Source: CAD feature listing. Evaluate the final solid. Frame: model axes, mm. Face numbers are marked on the shaded views. Round coordinates to 2 decimals unless told otherwise and drop trailing zeros. Loops run counter-clockwise (first coordinate to the right, second up) from the corner with the lowest first, then second, coordinate; pieces in that order, holes last. Notation, with made-up numbers: (8.25, 10) - (49.25, 10) arc R17 ccw to (49.25, 23) - close; hole circle Ø3 at (75, 87.25). An arc over 180 degrees is marked (long way). One line per question, with ' | ' between items. Start each with the question number.
1. Ray query, line 1 (Y direction, x = 12, z = 278.5); line 2 (X direction, y = 19, z = 761.5); line 3 (X direction, y = 4.3, z = 390). Return the intervals inside material, ascending.
2. Cut plane A-A (x = 25). Return loops of the section in (y, z), then the cut area to 3 significant figures.
3. Cut plane C-C (y = 57). Return loops of the section in (x, z) (3 decimals), then the cut area to 3 significant figures.
4. Cut plane D-D (z = 1113.5). Return loops of the section in (x, y).
5. Mould query, pull axis X, two halves, no side actions, for the marked faces 1 and 2. Classes: pulls with the +X half, pulls with the -X half, needs draft (parallel to the pull), parting line crosses it, or undercut.
6. Cut plane B-B (z = 303). Return loops of the section in (x, y), then the cut area to 3 significant figures.
7. Pin query (flat end, axial travel): pin 1 (4 mm diameter, centred on x = 10, z = 354, fed in from -Y); pin 2 (1 mm diameter, centred on y = 2.5, z = 469.5, fed in from -X); pin 3 (10 mm diameter, centred on y = -6, z = 932, fed in from +X); pin 4 (3 mm diameter, centred on x = 39, z = 341.5, fed in from -Y). Return the tip coordinate at first contact, or that it passes through.
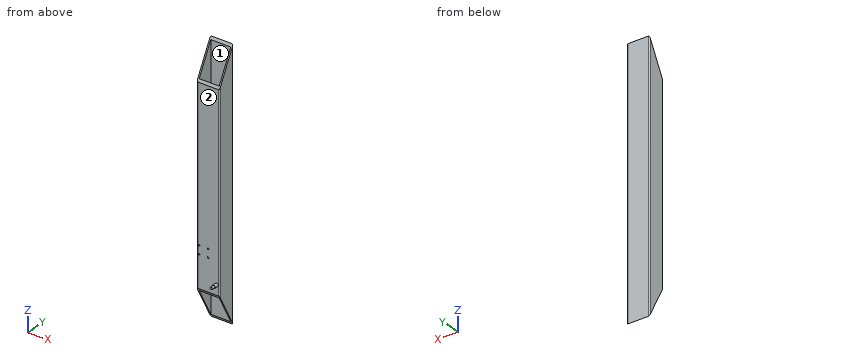
```python
from build123d import *

# Parameters (mm, degrees)
SCHIZZO1_W                   = 88
SCHIZZO1_H                   = 68
ESTRUSIONE_SOTTILE1_DEPTH    = 1200
ESTRUSIONE1_DEPTH            = 1207.813987324
SCHIZZO3_R                   = 3.4
TAGLIO_ESTRUSIONE1_DEPTH     = 10
RIPETIZIONE_A_L1_COUNT       = 2
RIPETIZIONE_A_L1_PITCH       = 40
RIPETIZIONE_A_L1_COUNT_DIR2  = 2
RIPETIZIONE_A_L1_PITCH_DIR2  = 36
SCHIZZO4_R                   = 7
ESTRUSIONE_ESTRUSIONE1_DEPTH = 18
SCHIZZO5_R                   = 5
ESTRUSIONE_ESTRUSIONE2_DEPTH = 15


with BuildPart() as part:
    # Schizzo1 → Estrusione-Sottile1 (new body)
    with BuildSketch(Plane.XY):
        with BuildLine():
            Line((5, 0), (95, 0))
            ThreePointArc((95, 0), (98.535533906, 1.464466094), (100, 5))
            Line((100, 5), (100, 75))
            ThreePointArc((100, 75), (98.535533906, 78.535533906), (95, 80))
            Line((95, 80), (5, 80))
            ThreePointArc((5, 80), (1.464466094, 78.535533906), (0, 75))
            Line((0, 75), (0, 5))
            ThreePointArc((0, 5), (1.464466094, 1.464466094), (5, 0))
        make_face()
        with Locations((50, 40)):
            Rectangle(SCHIZZO1_W, SCHIZZO1_H, mode=Mode.SUBTRACT)
    extrude(amount=ESTRUSIONE_SOTTILE1_DEPTH)

    # Schizzo2 → Estrusione1 (cut, through all)
    with BuildSketch(Plane(origin=(100, 0, 0), x_dir=(0, 0, -1), z_dir=(1, 0, 0))):
        Polygon((-1200, 80), (-1050, 0), (-1200, 0), align=None)
        Polygon((-64, 80), (-214, 0), (0, 0), (0, 80), align=None)
    extrude(amount=-ESTRUSIONE1_DEPTH, mode=Mode.SUBTRACT)

    # Schizzo3 → Taglio-Estrusione1 (cut)
    with BuildSketch(Plane.XZ):
        with Locations(Location((10, 354, 0), (0, 0, 270))):
            Circle(SCHIZZO3_R)
    taglio_estrusione1 = extrude(amount=-TAGLIO_ESTRUSIONE1_DEPTH, mode=Mode.SUBTRACT)

    # Ripetizione a L1: Taglio-Estrusione1 2 × 2
    with Locations(*[(i * RIPETIZIONE_A_L1_PITCH, 0, j * RIPETIZIONE_A_L1_PITCH_DIR2) for i in range(RIPETIZIONE_A_L1_COUNT) for j in range(RIPETIZIONE_A_L1_COUNT_DIR2) if (i, j) != (0, 0)]):
        add(taglio_estrusione1, mode=Mode.SUBTRACT)

    # Schizzo4 → Estrusione-Estrusione1 (add)
    with BuildSketch(Plane.XZ):
        with Locations((88, 257)):
            Circle(SCHIZZO4_R)
    extrude(amount=ESTRUSIONE_ESTRUSIONE1_DEPTH)

    # Schizzo5 → Estrusione-Estrusione2 (add)
    with BuildSketch(Plane.XZ.offset(18)):
        with Locations(Location((88, 257, 0), (0, 0, 270))):
            Circle(SCHIZZO5_R)
    extrude(amount=ESTRUSIONE_ESTRUSIONE2_DEPTH)


solid = part.part
```
Answers follow:
1) line 1: y = 0 to 6, 74 to 80 | line 2: x = 0 to 6, 94 to 100 | line 3: x = 0.05 to 6.6, 13.4 to 46.6, 53.4 to 99.95
2) outline: (0, 214) - (6, 202.75) - (6, 1061.25) - (0, 1050) - close; (74, 75.25) - (80, 64) - (80, 1200) - (74, 1188.75) - close | area: 11,800 mm2
3) outline: (0, 107.125) - (6, 107.125) - (6, 1156.875) - (0, 1156.875) - close; (94, 107.125) - (100, 107.125) - (100, 1156.875) - (94, 1156.875) - close | area: 12,600 mm2
4) outline: (0, 33.87) - (6, 33.87) - (6, 74) - (94, 74) - (94, 33.87) - (100, 33.87) - (100, 75) arc R5 ccw to (95, 80) - (5, 80) arc R5 ccw to (0, 75) - close
5) face 1: undercut | face 2: needs draft
6) outline: (0, 5) arc R5 ccw to (5, 0) - (95, 0) arc R5 ccw to (100, 5) - (100, 75) arc R5 ccw to (95, 80) - (5, 80) arc R5 ccw to (0, 75) - close; hole (6, 6) - (94, 6) - (94, 74) - (6, 74) - close | area: 1,990 mm2
7) pin 1: stops at y = 74 | pin 2: stops at x = 0.42 | pin 3: passes through | pin 4: stops at y = 0
